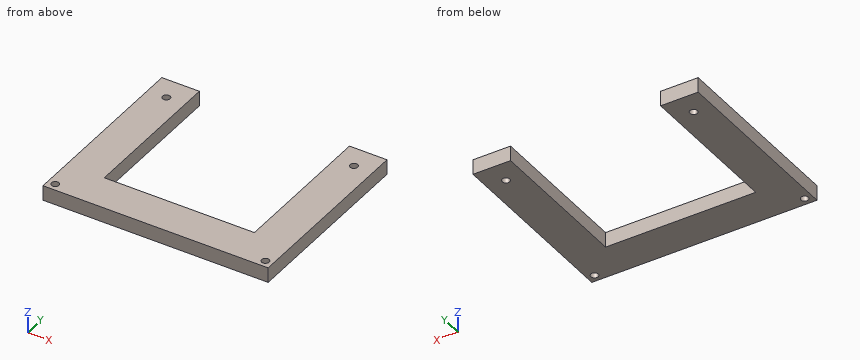
from build123d import *

# Parameters (mm, degrees)
BOSS_EXTRUDE1_DEPTH = 20
CUT_EXTRUDE1_REACH  = 393.024
SKETCH2_R           = 5
CUT_EXTRUDE2_REACH  = 393.024
SKETCH3_R           = 5


with BuildPart() as part:
    # Sketch1 → Boss-Extrude1 (new body)
    with BuildSketch(Plane.XY):
        Polygon((0, 0), (0, -250), (300, -250), (300, 0), (250, 0), (250, -200), (50, -200), (50, 0), align=None)
    extrude(amount=BOSS_EXTRUDE1_DEPTH)

    # Sketch2 → Cut-Extrude1 (cut, up to next)
    with BuildSketch(Plane.XY.offset(20), mode=Mode.PRIVATE) as cut_extrude1_sk1:
        with Locations((25, -30)):
            Circle(SKETCH2_R)
    cut_extrude1_tool1 = extrude(cut_extrude1_sk1.sketch, amount=-CUT_EXTRUDE1_REACH, mode=Mode.PRIVATE) & part.part
    # Sketch2 → Cut-Extrude1 (cut, up to next)
    with BuildSketch(Plane.XY.offset(20), mode=Mode.PRIVATE) as cut_extrude1_sk2:
        with Locations((275, -30)):
            Circle(SKETCH2_R)
    cut_extrude1_tool2 = extrude(cut_extrude1_sk2.sketch, amount=-CUT_EXTRUDE1_REACH, mode=Mode.PRIVATE) & part.part
    add(cut_extrude1_tool1.solids().sort_by_distance((25, -30, 20))[0], mode=Mode.SUBTRACT)
    add(cut_extrude1_tool2.solids().sort_by_distance((275, -30, 20))[0], mode=Mode.SUBTRACT)

    # Sketch3 → Cut-Extrude2 (cut, up to next)
    with BuildSketch(Plane(origin=(0, 0, 0), x_dir=(-1, 0, 0), z_dir=(0, 0, -1)), mode=Mode.PRIVATE) as cut_extrude2_sk1:
        with Locations((-290, -240)):
            Circle(SKETCH3_R)
    cut_extrude2_tool1 = extrude(cut_extrude2_sk1.sketch, amount=-CUT_EXTRUDE2_REACH, mode=Mode.PRIVATE) & part.part
    # Sketch3 → Cut-Extrude2 (cut, up to next)
    with BuildSketch(Plane(origin=(0, 0, 0), x_dir=(-1, 0, 0), z_dir=(0, 0, -1)), mode=Mode.PRIVATE) as cut_extrude2_sk2:
        with Locations(Location((-10, -240, 0), (0, 0, 180))):
            Circle(SKETCH3_R)
    cut_extrude2_tool2 = extrude(cut_extrude2_sk2.sketch, amount=-CUT_EXTRUDE2_REACH, mode=Mode.PRIVATE) & part.part
    add(cut_extrude2_tool1.solids().sort_by_distance((290, -240, 0))[0], mode=Mode.SUBTRACT)
    add(cut_extrude2_tool2.solids().sort_by_distance((10, -240, 0))[0], mode=Mode.SUBTRACT)


solid = part.part
Input: part model. Units: mm. Frame: model coordinates. Coordinates: 2 decimals unless noted, no trailing zeros. Loops run counter-clockwise (first coordinate to the right, second up) from the corner with the lowest first, then second, coordinate; pieces in that order, holes last.
(1) Section C-C on z = 7.75. Return the cut outline in (x, y), then the cut area to 3 significant figures.
(2) Section B-B on y = -30. Return the cut outline in (x, z).
(3) Section A-A on x = 290. Return the cut outline in (y, z).
(4) Material intervals for probe 1 along X at (y, z) = (-198.5, 13); probe 2 along Y at (x, z) = (25, 14.25); probe 3 along Y at (x, z) = (10, 12.25), sorted ascending.
(5) Section D-D on y = -132. Return the cut outline in (x, z), then the cut area to 3 significant figures.
(6) First-contact query: pin 1 Ø10 at (x, z) = (152.5, 6) entering from +Y. Flat tip, straight axial feed; report the tip coordinate or a pass-through.
Data:
1. outline: (0, -250) - (300, -250) - (300, 0) - (250, 0) - (250, -200) - (50, -200) - (50, 0) - (0, 0) - close; hole circle Ø10 at (10, -240); hole circle Ø10 at (25, -30); hole circle Ø10 at (275, -30); hole circle Ø10 at (290, -240)
1. area: 34,700 mm2
2. outline: (0, 0) - (20, 0) - (20, 20) - (0, 20) - close; (30, 0) - (50, 0) - (50, 20) - (30, 20) - close; (250, 0) - (270, 0) - (270, 20) - (250, 20) - close; (280, 0) - (300, 0) - (300, 20) - (280, 20) - close
3. outline: (-250, 0) - (-245, 0) - (-245, 20) - (-250, 20) - close; (-235, 0) - (0, 0) - (0, 20) - (-235, 20) - close
4. probe 1: x = 0 to 50, 250 to 300
4. probe 2: y = -250 to -35, -25 to 0
4. probe 3: y = -250 to -245, -235 to 0
5. outline: (0, 0) - (50, 0) - (50, 20) - (0, 20) - close; (250, 0) - (300, 0) - (300, 20) - (250, 20) - close
5. area: 2,000 mm2
6. pin 1: stops at y = -200
